The model under review builds one solid part; all positions refer to its coordinate system, in mm. A direction names the side the tool comes from. Round coordinates to 2 decimals unless told otherwise and drop trailing zeros. Loops run counter-clockwise (first coordinate to the right, second up) from the corner with the lowest first, then second, coordinate; pieces in that order, holes last. Notation, with made-up numbers: M 40,-36.5 L 64,-36.5 A20 cw 64,-26.5 Z; hole C 8,37.5 d11. An arc over 180 degrees is marked long. Use a Markdown table: item, result. Add a question column.
```python
from build123d import *

# Parameters (mm, degrees)
F1_DEPTH  = 5
F3_DEPTH  = 3
F5_DEPTH  = 3
F7_DEPTH  = 5
F8_R      = 2.49999
F9_R      = 1.5
F10_DEPTH = 5


# Not quite as in the source:
# - a fillet or chamfer is up to 0.001 mm smaller than in the source, because OpenCascade refuses the exact size


with BuildPart() as f1:
    # F0 (on Top) → F1 (new body)
    with BuildSketch(Plane.XY):
        Polygon((0, 6), (0, 0), (7.8194713464, -9.1025198634), (13.8194713464, -9.1025198634), (19.8194713464, -9.1025198634), (27.6389426928, 0), (27.6389426928, 6), (27.6389426928, 12), (19.8194713464, 21.1025198634), (13.8194713464, 21.1025198634), (7.8194713464, 21.1025198634), (0, 12), align=None)
    extrude(amount=F1_DEPTH)

    # F2 (on face) → F3 (cut)
    with BuildSketch(Plane.XY.offset(5)):
        Polygon((2, 11.2589063868), (2, 0.7410936132), (8.7380145007, -7.1025198634), (18.9009281921, -7.1025198634), (25.6389426928, 0.7410936132), (25.6389426928, 11.2589063868), (18.9009281921, 19.1025198634), (8.7380145007, 19.1025198634), align=None)
    extrude(amount=-F3_DEPTH, mode=Mode.SUBTRACT)

    # F4 (on face) → F5 (join)
    with BuildSketch(Plane.XY.offset(2)):
        Polygon((17.9823850378, -5.1025198634), (23.6389426928, 1.4821872264), (23.6389426928, 10.5178127736), (17.9823850378, 17.1025198634), (14.4432382658, 17.1025198634), (14.4432382658, -5.1025198634), align=None)
        Polygon((16.4432382658, -3.1025198634), (16.4432382658, 15.1025198634), (17.0638418835, 15.1025198634), (21.6389426928, 9.7767191605), (21.6389426928, 2.2232808395), (17.0638418835, -3.1025198634), align=None, mode=Mode.SUBTRACT)
        Polygon((10.7860844582, -3.1025198634), (10.7860844582, -5.1025198634), (12.7860844582, -5.1025198634), (12.7860844582, 17.1025198634), (9.6565576549, 17.1025198634), (4, 10.5178127736), (4, 1.4821872264), (6.8282788275, -1.8101663185), (8.3453654714, -0.5069210941), (6, 2.2232808395), (6, 5.4149306379), (10.7860844582, 5.4149306379), align=None)
        Polygon((6, 9.7767191605), (10.5751008092, 15.1025198634), (10.7860844582, 15.1025198634), (10.7860844582, 6.9169756025), (6, 6.9169756025), align=None, mode=Mode.SUBTRACT)
    extrude(amount=F5_DEPTH)

    # F6 (on face) → F7 (join)
    with BuildSketch(Plane(origin=(0, 21.1025198634, 0), x_dir=(-1, 0, 0), z_dir=(0, 1, 0))):
        Polygon((-11.3194713464, 5), (-13.8194713464, 5), (-16.3194713464, 5), (-16.3194713464, 0), (-11.3194713464, 0), align=None)
    extrude(amount=F7_DEPTH)

    # F8 (radius 2.5 in the source; OpenCascade refuses exactly that, so slightly less here)
    f8_edges = [f1.edges().sort_by_distance(p)[0] for p in [
        (11.319471, 26.10252, 2.5),
        (16.319471, 26.10252, 2.5),
    ]]
    fillet(f8_edges, radius=F8_R)

    # F9 (on face) → F10 (cut)
    with BuildSketch(Plane.XY.offset(5)):
        with Locations((13.8194713464, 23.6025198634)):
            Circle(F9_R)
    extrude(amount=-F10_DEPTH, mode=Mode.SUBTRACT)


solid = f1.part
```
(1) Consider section D-D, the plane y = -1. Give the boundary of the cut face in (x, z), then the cut area to 3 significant figures.
(2) Consider section A-A, the plane y = 23. Give the boundary of the cut face in (x, z), then the cut area to 3 significant figures.
(3) To check wall thickness, follow probe 1 along Y at (x, z) = (11, 3); probe 2 along Y at (x, z) = (17.75, 4.5); probe 3 along X at (y, z) = (0, 4.55). State the ranges of each line that lie inside material, in increasing order.
(4) Consider section B-B, the plane z = 3.55. Give the number of separate pieces and of enclosed holes in the cut face, then the cut area to 3 significant figures.
(5) For faces 1 (the face through (18, 21.103, 2)), 2 (the face through (6, 8, 3)), 3 (the face through (11.319, 22, 2)), 4 (the face through (15.205, 23.028, 2.535)), 5 (the face through (24, 14, 5)), list the 3-axis set-ups (+Z, -Z, +X, -X, +Y, -Y) from which the entire face can be reached by the end or side of a thin tool; tool diameter is ignored.
(6) Insertion check: pin 1 Ø1 at (y, z) = (21.5, 0.5) entering from -X; pin 2 Ø2 at (y, z) = (22, 2.5) entering from +X; pin 3 Ø2.5 at (x, z) = (16.5, 3.5) entering from +Y. Each pin has a flat end and moves straight along its axis. Give the tip position at first contact, or say it passes through.
Found:
| question | item | result |
|---|---|---|
| 1 | outline | M 0.86,0 L 26.78,0 L 26.78,5 L 24.14,5 L 24.14,2 L 21.51,2 L 21.51,5 L 18.87,5 L 18.87,2 L 16.44,2 L 16.44,5 L 14.44,5 L 14.44,2 L 12.79,2 L 12.79,5 L 10.79,5 L 10.79,2 L 7.77,2 L 7.77,5 L 6.13,5 L 6.13,2 L 3.5,2 L 3.5,5 L 0.86,5 Z |
| 1 | area | 92.5 mm^2 |
| 2 | outline | M 11.32,0 L 12.45,0 L 12.45,5 L 11.32,5 Z; M 15.19,0 L 16.32,0 L 16.32,5 L 15.19,5 Z |
| 2 | area | 11.3 mm^2 |
| 3 | probe 1 | y = -9.1 to -7.1, -5.1 to 17.1, 19.1 to 21.1 |
| 3 | probe 2 | y = -9.1 to -7.1, -5.1 to -2.3, 14.3 to 17.1, 19.1 to 21.1 |
| 3 | probe 3 | x = 0 to 2.64, 5.27 to 7.91, 10.79 to 12.79, 14.44 to 16.44, 19.73 to 22.37, 25 to 27.64 |
| 4 | separate pieces | 3 |
| 4 | enclosed holes | 4 |
| 4 | area | 384 mm^2 |
| 5 | face 1 | +Z, -Z, +X, +Y |
| 5 | face 2 | +Z |
| 5 | face 3 | +Z, -Z, -X, +Y |
| 5 | face 4 | +Z, -Z |
| 5 | face 5 | +Z, +X, -X, +Y, -Y |
| 6 | pin 1 | stops at x = 7.73 |
| 6 | pin 2 | stops at x = 19.91 |
| 6 | pin 3 | stops at y = 25.65 |
